Verification items for this drawing (mm, ordinates from the low corner). A direction names the side the tool comes from. Coordinates: 2 decimals unless noted, no trailing zeros. Write each loop counter-clockwise with the first axis right and the second up, starting at its lowest first coordinate (ties: lowest second). Pieces come first, ordered by that corner, then holes. Notation, with made-up numbers: (27.5, 80) -> (48.5, 80) arc R31 cw to (48.5, 106) -> close; hole circle Ø5 at (41, 74). An arc over 180 degrees is marked (long way). Answer as CSV lines item,"result".
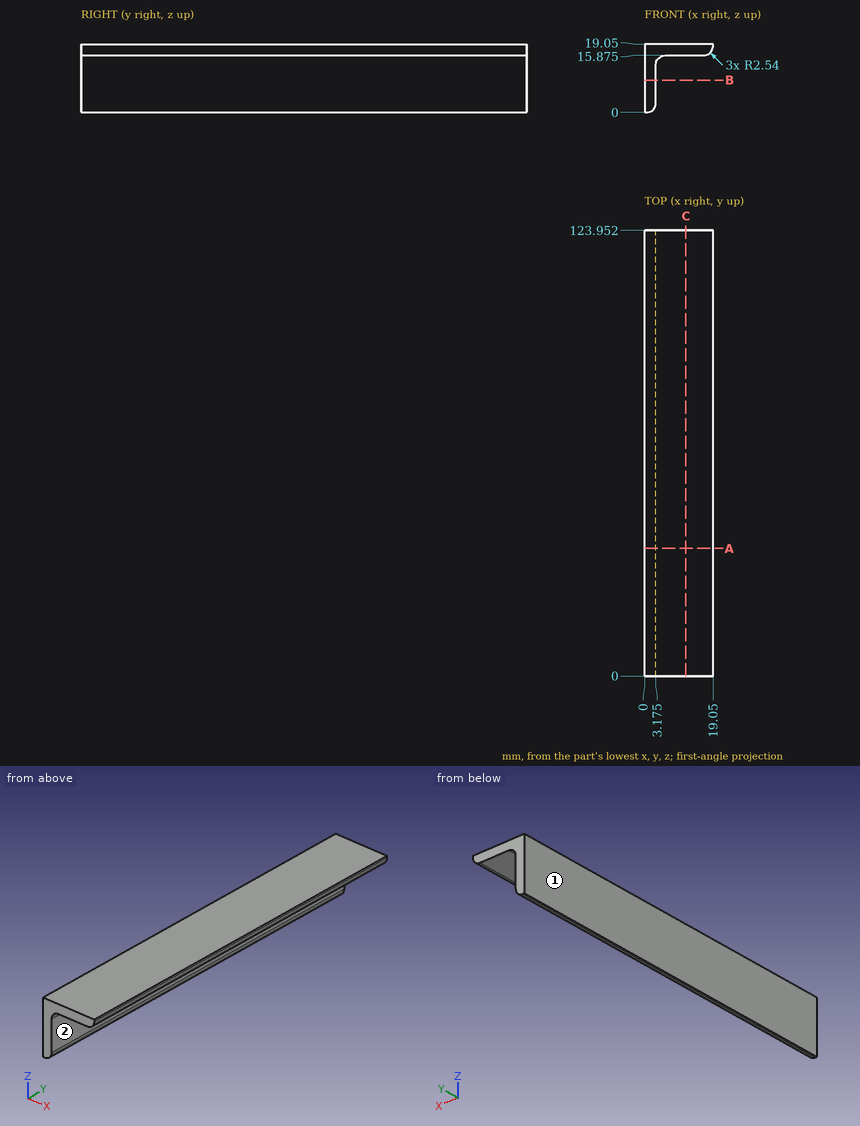
Item 1: Cross-section at C-C, the plane x = 11.5. Record the cut outline in (y, z) (3 decimals).
Responses:
outline,"(0, 15.875) -> (123.952, 15.875) -> (123.952, 19.05) -> (0, 19.05) -> close"
Item 2: Cross-section at A-A, the plane y = 35.5. Record the cut outline in (x, z) (3 decimals).
Responses:
outline,"(0, 0) -> (0.635, 0) arc R2.54 ccw to (3.175, 2.54) -> (3.175, 13.335) arc R2.54 cw to (5.715, 15.875) -> (16.51, 15.875) arc R2.54 ccw to (19.05, 18.415) -> (19.05, 19.05) -> (0, 19.05) -> close"
Item 3: Cross-section at B-B, the plane z = 9. Record the cut outline in (x, y) (3 decimals).
Responses:
outline,"(0, 0) -> (3.175, 0) -> (3.175, 123.952) -> (0, 123.952) -> close"
Item 4: Thickness scan on probe 1 along X at (y, z) = (15, 5.5) (3 decimals); probe 2 along Z at (x, y) = (7, 68) (3 decimals); probe 3 along Z at (x, y) = (17.5, 82). Record the ranges inside material, lowest first.
Responses:
probe 1,"x = 0 to 3.175"
probe 2,"z = 15.875 to 19.05"
probe 3,"z = 16.08 to 19.05"
Item 5: Set-up check for the marked faces 1 and 2: record each of +Z, -Z, +X, -X, +Y, -Y from which the full face is reachable in a straight line by a thin tool's end or side.
Responses:
face 1,"+Z, -Z, -X, +Y, -Y"
face 2,"-Z, +X, +Y, -Y"
Item 6: Depth check by flat-ended pin: pin 1 Ø1 at (y, z) = (72.5, 13) entering from +X; pin 2 Ø5.5 at (x, y) = (12, 38) entering from -Z (3 decimals). Enter the tip coordinate at first touch or a pass-through.
Responses:
pin 1,"stops at x = 3.18"
pin 2,"stops at z = 15.875"
